Design review of the part shown in the three views and the two pictorial views. Dimensions are in mm from the part's minimum x, y and z. A direction names the side the tool comes from. Coordinates: 2 decimals unless noted, no trailing zeros. Write each loop counter-clockwise with the first axis right and the second up, starting at its lowest first coordinate (ties: lowest second). Pieces come first, ordered by that corner, then holes.
Q1. For pin 1 Ø12 at (x, y) = (42.5, 25.5) entering from -Z; pin 2 Ø2.5 at (x, z) = (37.5, 16) entering from +Y; pin 3 Ø1.5 at (y, z) = (43, 11) entering from +X; pin 4 Ø5.5 at (x, z) = (39.5, 15) entering from -Y, all flat-tipped, find the tip position at first contact; note any pin that passes through.
Q2. Take a section at C-C, the plane z = 12.75. State how many separate pieces and enclosed holes the cut face has, plus the area to 3 significant figures.
Q3. Take a section at B-B, the plane z = 18.75. Write out the cut boundary in (x, y), plus the area to 3 significant figures.
Q4. For L1, parallel to X at y = 7.1, z = 20.75; L2, parallel to Z at x = 38.5, y = 41.9; L3, parallel to Y at x = 25, z = 3, list the stretches that pass through material, from the lowest coordinate up.
Q5. Take a section at D-D, the plane x = 17. Write out the cut boundary in (y, z), plus the area to 3 significant figures.
Q6. For the marked faces 1, 2, 3 and 4, list the 3-axis set-ups (+Z, -Z, +X, -X, +Y, -Y) from which the entire face can be reached by the end or side of a thin tool; tool diameter is ignored.
Q7. Take a section at A-A, the plane x = 25. Write out the cut boundary in (y, z), plus the area to 3 significant figures.
Q8. The part is to be moulded in two halves that separate along Y. For the marked faces 5, 6 and 7, say which applies: released by +Y, released by -Y, zero draft, split by the parting line, or undercut.
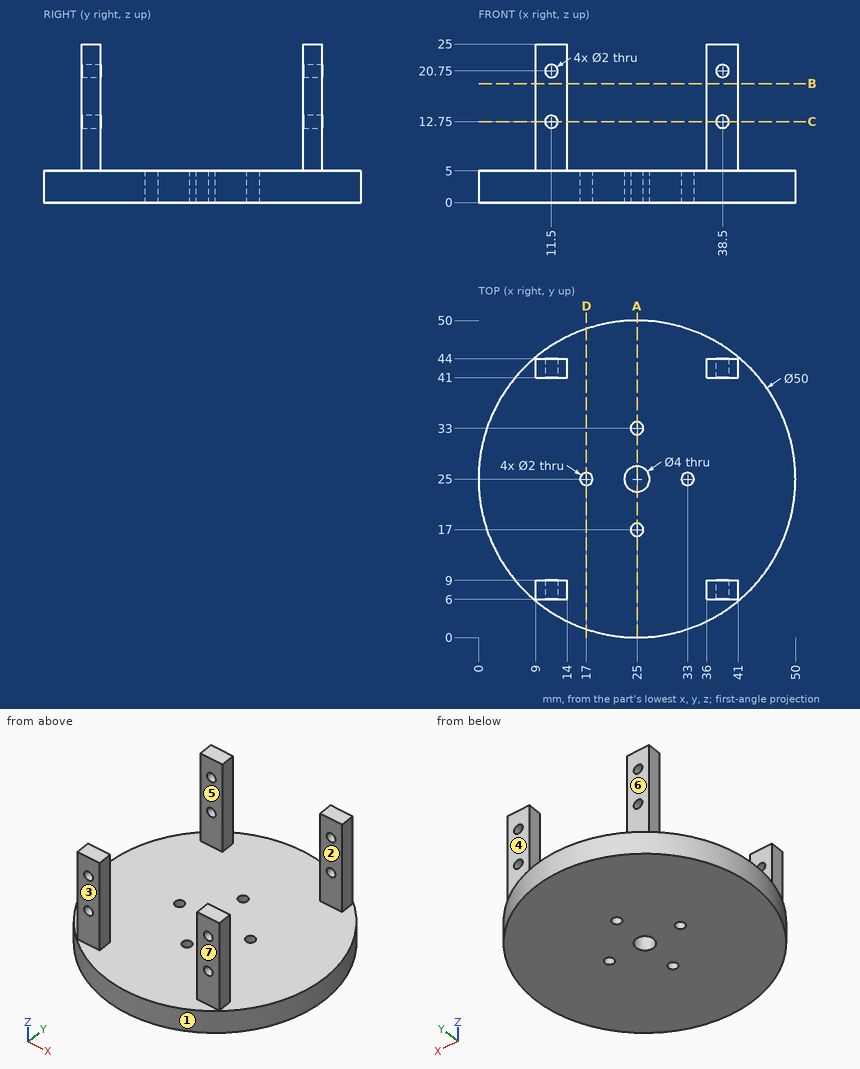
Responses:
1. pin 1: stops at z = 0
1. pin 2: stops at y = 44
1. pin 3: stops at x = 41
1. pin 4: stops at y = 6
2. separate pieces: 8
2. enclosed holes: 0
2. area: 36.0 mm2
3. outline: (9, 6) - (14, 6) - (14, 9) - (9, 9) - close; (9, 41) - (14, 41) - (14, 44) - (9, 44) - close; (36, 6) - (41, 6) - (41, 9) - (36, 9) - close; (36, 41) - (41, 41) - (41, 44) - (36, 44) - close
3. area: 60.0 mm2
4. L1: x = 9 to 10.5, 12.5 to 14, 36 to 37.5, 39.5 to 41
4. L2: z = 0 to 11.75, 13.75 to 19.75, 21.75 to 25
4. L3: y = 0 to 16, 18 to 23, 27 to 32, 34 to 50
5. outline: (1.31, 0) - (24, 0) - (24, 5) - (1.31, 5) - close; (26, 0) - (48.69, 0) - (48.69, 5) - (26, 5) - close
5. area: 227 mm2
6. face 1: +Z, -Z
6. face 2: +Z, +X, -X
6. face 3: +Z, +X, -X, -Y
6. face 4: +Z, +X, -X, +Y
7. outline: (0, 0) - (16, 0) - (16, 5) - (0, 5) - close; (18, 0) - (23, 0) - (23, 5) - (18, 5) - close; (27, 0) - (32, 0) - (32, 5) - (27, 5) - close; (34, 0) - (50, 0) - (50, 5) - (34, 5) - close
7. area: 210 mm2
8. face 5: undercut
8. face 6: released by +Y
8. face 7: released by -Y
